Design review of the part built by this model. Coordinates are the model's own, in mm. A direction names the side the tool comes from. Round coordinates to 2 decimals unless told otherwise and drop trailing zeros. Loops run counter-clockwise (first coordinate to the right, second up) from the corner with the lowest first, then second, coordinate; pieces in that order, holes last. Notation, with made-up numbers: (17, -27.75) -> (25, -27.75) arc R20 ccw to (25, 0.25) -> close; hole circle Ø5 at (-1, 80.25). An arc over 180 degrees is marked (long way). Write each question's results on one line, items separated by ' | '. Start each with the question number.
from build123d import *

# Parameters (mm, degrees)
BOSS_EXTRUDE1_DEPTH = 5.5
CUT_EXTRUDE1_DEPTH  = 3
SKETCH3_W           = 7.5
SKETCH3_H           = 7.5
CUT_EXTRUDE2_DEPTH  = 0.5
SKETCH4_R           = 1.825
CUT_EXTRUDE3_DEPTH  = 10
SKETCH5_W           = 2.5
SKETCH5_H           = 8
CUT_EXTRUDE4_DEPTH  = 3
SKETCH6_W           = 7
SKETCH6_H           = 7
SKETCH6_R           = 1.825
BOSS_EXTRUDE2_DEPTH = 2.5
BOSS_EXTRUDE3_DEPTH = 1
CUT_EXTRUDE6_DEPTH  = 4
SKETCH10_W          = 12
SKETCH10_H          = 2.5
CUT_EXTRUDE7_DEPTH  = 4
CUT_EXTRUDE8_DEPTH  = 3


with BuildPart() as part:
    # Sketch1 → Boss-Extrude1 (new body)
    with BuildSketch(Plane(origin=(0, 0, 0), x_dir=(1, 0, 0), z_dir=(0, 1, 0))):
        with BuildLine():
            Line((-17.1, -15.5), (17.1, -15.5))
            ThreePointArc((17.1, -15.5), (18.514213562, -14.914213562), (19.1, -13.5))
            Line((19.1, -13.5), (19.1, 13.5))
            ThreePointArc((19.1, 13.5), (18.514213562, 14.914213562), (17.1, 15.5))
            Line((17.1, 15.5), (-17.1, 15.5))
            ThreePointArc((-17.1, 15.5), (-18.514213562, 14.914213562), (-19.1, 13.5))
            Line((-19.1, 13.5), (-19.1, -13.5))
            ThreePointArc((-19.1, -13.5), (-18.514213562, -14.914213562), (-17.1, -15.5))
        make_face()
    extrude(amount=BOSS_EXTRUDE1_DEPTH)

    # Sketch2 → Cut-Extrude1 (cut)
    with BuildSketch(Plane(origin=(0, 5.5, 0), x_dir=(1, 0, 0), z_dir=(0, 1, 0))):
        Polygon((-16.6, 5.5), (-9.1, 5.5), (-9.1, 13), (9.1, 13), (9.1, 5.5), (16.6, 5.5), (16.6, -5.5), (9.1, -5.5), (9.1, -13), (-9.1, -13), (-9.1, -5.5), (-16.6, -5.5), align=None)
    extrude(amount=-CUT_EXTRUDE1_DEPTH, mode=Mode.SUBTRACT)

    # Sketch3 → Cut-Extrude2 (cut)
    with BuildSketch(Plane(origin=(0, 5.5, 0), x_dir=(1, 0, 0), z_dir=(0, 1, 0))):
        with Locations((-12.85, 9.25)):
            Rectangle(SKETCH3_W, SKETCH3_H)
        with Locations((12.85, 9.25)):
            Rectangle(SKETCH3_W, SKETCH3_H)
        with Locations((12.85, -9.25)):
            Rectangle(SKETCH3_W, SKETCH3_H)
        with Locations((-12.85, -9.25)):
            Rectangle(SKETCH3_W, SKETCH3_H)
    extrude(amount=-CUT_EXTRUDE2_DEPTH, mode=Mode.SUBTRACT)

    # Sketch4 → Cut-Extrude3 (cut)
    with BuildSketch(Plane(origin=(0, 5.5, 0), x_dir=(1, 0, 0), z_dir=(0, 1, 0))):
        with Locations(Location((-12.425, 8.675, 0), (0, 0, 270))):
            Circle(SKETCH4_R)
        with Locations(Location((12.425, 8.675, 0), (0, 0, 90))):
            Circle(SKETCH4_R)
        with Locations(Location((12.425, -8.675, 0), (0, 0, 270))):
            Circle(SKETCH4_R)
        with Locations(Location((-12.425, -8.675, 0), (0, 0, 270))):
            Circle(SKETCH4_R)
    extrude(amount=-CUT_EXTRUDE3_DEPTH, mode=Mode.SUBTRACT)

    # Sketch5 → Cut-Extrude4 (cut)
    with BuildSketch(Plane(origin=(0, 5.5, 0), x_dir=(1, 0, 0), z_dir=(0, 1, 0))):
        with Locations((-17.85, -1.5)):
            Rectangle(SKETCH5_W, SKETCH5_H)
        with Locations((17.85, -1.5)):
            Rectangle(SKETCH5_W, SKETCH5_H)
    extrude(amount=-CUT_EXTRUDE4_DEPTH, mode=Mode.SUBTRACT)

    # Sketch6 → Boss-Extrude2 (add)
    # profile 1 of 2: a face of its own
    with BuildSketch(Plane(origin=(0, 0, 0), x_dir=(1, 0, 0), z_dir=(0, 1, 0))):
        with Locations((-0.35, 19)):
            Rectangle(SKETCH6_W, SKETCH6_H)
        with Locations(Location((-0.35, 19, 0), (0, 0, 270))):
            Circle(SKETCH6_R, mode=Mode.SUBTRACT)
    # profile 2 of 2: a face of its own
    with BuildSketch(Plane(origin=(0, 0, 0), x_dir=(1, 0, 0), z_dir=(0, 1, 0))):
        with Locations((-0.35, -19)):
            Rectangle(SKETCH6_W, SKETCH6_H)
        with Locations(Location((-0.35, -19, 0), (0, 0, 90))):
            Circle(SKETCH6_R, mode=Mode.SUBTRACT)
    extrude(amount=BOSS_EXTRUDE2_DEPTH)

    # Sketch7 → Boss-Extrude3 (add)
    with BuildSketch(Plane(origin=(0, 5.5, 0), x_dir=(1, 0, 0), z_dir=(0, 1, 0))):
        with BuildLine():
            ThreePointArc((-17.1, -14.15), (-17.559619408, -13.959619408), (-17.75, -13.5))
            Line((-17.75, -13.5), (-17.75, -5.5))
            Line((-17.75, -5.5), (-16.6, -5.5))
            Line((-16.6, -5.5), (-16.6, -13))
            Line((-16.6, -13), (16.6, -13))
            Line((16.6, -13), (16.6, -5.5))
            Line((16.6, -5.5), (17.75, -5.5))
            Line((17.75, -5.5), (17.75, -13.5))
            ThreePointArc((17.75, -13.5), (17.559619408, -13.959619408), (17.1, -14.15))
            Line((17.1, -14.15), (-17.1, -14.15))
        make_face()
        with BuildLine():
            Line((16.6, 2.5), (17.75, 2.5))
            Line((17.75, 2.5), (17.75, 13.5))
            ThreePointArc((17.75, 13.5), (17.559619408, 13.959619408), (17.1, 14.15))
            Line((17.1, 14.15), (-17.1, 14.15))
            ThreePointArc((-17.1, 14.15), (-17.559619408, 13.959619408), (-17.75, 13.5))
            Line((-17.75, 13.5), (-17.75, 2.5))
            Line((-17.75, 2.5), (-16.6, 2.5))
            Line((-16.6, 2.5), (-16.6, 13))
            Line((-16.6, 13), (16.6, 13))
            Line((16.6, 13), (16.6, 2.5))
        make_face()
    extrude(amount=BOSS_EXTRUDE3_DEPTH)

    # Sketch9 → Cut-Extrude6 (cut)
    with BuildSketch(Plane(origin=(0, 0, -15.5), x_dir=(-1, 0, 0), z_dir=(0, 0, -1))):
        with BuildLine():
            Line((5.1, 4), (-3.9, 4))
            ThreePointArc((-3.9, 4), (-5.4, 5.5), (-3.9, 7))
            Line((-3.9, 7), (5.1, 7))
            ThreePointArc((5.1, 7), (6.6, 5.5), (5.1, 4))
        make_face()
    extrude(amount=-CUT_EXTRUDE6_DEPTH, mode=Mode.SUBTRACT)

    # Sketch10 → Cut-Extrude7 (cut)
    with BuildSketch(Plane(origin=(0, 5.5, 0), x_dir=(1, 0, 0), z_dir=(0, 1, 0))):
        with Locations((-0.6, 14.25)):
            Rectangle(SKETCH10_W, SKETCH10_H)
    extrude(amount=CUT_EXTRUDE7_DEPTH, mode=Mode.SUBTRACT)

    # Sketch12 → Cut-Extrude8 (cut)
    with BuildSketch(Plane.XZ):
        Polygon((-12.425, 12.139101615), (-15.425, 10.407050808), (-15.425, 6.942949192), (-12.425, 5.210898385), (-9.425, 6.942949192), (-9.425, 10.407050808), align=None)
        Polygon((9.425, 10.407050808), (12.425, 12.139101615), (15.425, 10.407050808), (15.425, 6.942949192), (12.425, 5.210898385), (9.425, 6.942949192), align=None)
        Polygon((12.425, -12.139101615), (15.425, -10.407050808), (15.425, -6.942949192), (12.425, -5.210898385), (9.425, -6.942949192), (9.425, -10.407050808), align=None)
        Polygon((-9.425, -10.407050808), (-12.425, -12.139101615), (-15.425, -10.407050808), (-15.425, -6.942949192), (-12.425, -5.210898385), (-9.425, -6.942949192), align=None)
    extrude(amount=-CUT_EXTRUDE8_DEPTH, mode=Mode.SUBTRACT)


solid = part.part
1) Take a section at B-B (z = -19). Write out the cut boundary in (x, y) (3 decimals), plus the area to 4 significant figures.
2) To check wall thickness, follow line 1 (X direction, y = 1.5, z = 9.5) (3 decimals); line 2 (X direction, y = 5.25, z = -12); line 3 (X direction, y = 0.75, z = 12). State the ranges of each line that lie inside material, in increasing order. Write a range as from..to.
3) Insertion check: pin 1 (0.8 mm diameter, centred on x = 1.5, z = -13.5, fed in from +Y); pin 2 (5 mm diameter, centred on x = -4, z = -8, fed in from +Y); pin 3 (0.5 mm diameter, centred on y = 6, z = -13.5, fed in from +X); pin 4 (1.2 mm diameter, centred on y = 6, z = 9.5, fed in from -X). Each pin has a flat end and moves straight along its axis. Give the tip position at first contact, or say it passes through.
4) Take a section at A-A (x = -0.35). Write out the cut boundary in (y, z) (3 decimals).
5) For faces 1 (the face through (9.1, 4, 9)), 2 (the face through (13.904, 1.479, -11.285)), 3 (the face through (-3.85, 1, -19)), 4 (the face through (-1, 4, -14)), 5 (the face through (-17.75, 6, 10)), list the 3-axis set-ups (+Z, -Z, +X, -X, +Y, -Y) from which the entire face can be reached by the end or side of a thin tool; tool diameter is ignored.
6) Take a section at C-C (y = 4.5). State how many separate pieces and enclosed holes the cut face has, plus the area to 3 significant figures.
Geometry check:
1) outline: (-3.85, 0) -> (-2.175, 0) -> (-2.175, 2.5) -> (-3.85, 2.5) -> close; (1.475, 0) -> (3.15, 0) -> (3.15, 2.5) -> (1.475, 2.5) -> close | area: 8.375 mm^2
2) line 1: x = -19.1..-15.425, -9.425..9.425, 15.425..19.1 | line 2: x = -19.1..-16.6, 16.6..19.1 | line 3: x = -19.1..-12.67, -12.18..12.18, 12.67..19.1
3) pin 1: stops at y = 4 | pin 2: stops at y = 2.5 | pin 3: stops at x = 17.75 | pin 4: stops at x = -19.1
4) outline: (0, -22.5) -> (2.5, -22.5) -> (2.5, -20.825) -> (0, -20.825) -> close; (0, -17.175) -> (2.5, -17.175) -> (2.5, -15.5) -> (4, -15.5) -> (4, -13) -> (2.5, -13) -> (2.5, 13) -> (6.5, 13) -> (6.5, 14.15) -> (5.5, 14.15) -> (5.5, 15.5) -> (2.5, 15.5) -> (2.5, 17.175) -> (0, 17.175) -> close; (0, 20.825) -> (2.5, 20.825) -> (2.5, 22.5) -> (0, 22.5) -> close
5) face 1: +Y | face 2: -Y | face 3: -Z, -X, +Y, -Y | face 4: -Z, +Y | face 5: +Z, -Z, -X, +Y
6) separate pieces: 3 | enclosed holes: 4 | area: 433 mm^2
